Autodesk Inventor part; units mm, degrees
ref_plane "YZ Plane" through (0, 0, 0) normal (1, 0, 0) x (0, 1, 0)
ref_plane "XZ Plane" through (0, 0, 0) normal (0, 1, 0) x (-1, 0, 0)
ref_plane "XY Plane" through (0, 0, 0) normal (0, 0, 1) x (1, 0, 0)
sketch "Sketch1" plane through (0, 0, 0) normal (0, 0, 1) x (1, 0, 0)
  circle A0 centre (0, 0) radius 1.5
  arc A1 (-0.6702, -11.9813) -> (0, 12) centre (0, 0) ccw
  circle A2 centre (-50, 0) radius 1.5
  arc A3 (-6.6581, 4.4351) -> (-6.6581, -4.4351) centre (0, 0) ccw
  line L0 (-44.9603, 5.4977) -> (-8.4343, 7.5407)
  line L1 (-44.9603, -5.4977) -> (-8.4343, -7.5407)
  arc A4 (-44.9603, 5.4977) -> (-46.0589, 3.0769) centre (-44.8765, 4) ccw
  arc A5 (-46.0589, -3.0769) -> (-44.9603, -5.4977) centre (-44.8765, -4) ccw
  arc A6 (-6.6581, 4.4351) -> (-8.4343, 7.5407) centre (-8.3226, 5.5439) ccw
  arc A7 (-8.4343, -7.5407) -> (-6.6581, -4.4351) centre (-8.3226, -5.5439) ccw
  line L2 (-104, 0) -> (-57, 0) construction
  line L3 (-106, -18) -> (-104, -18)
  line L4 (-98, -12) -> (-98, -6.6741)
  line L5 (-112, -12) -> (-112, 18)
  arc A8 (-94.8953, -3.6759) -> (-98, -6.6741) centre (-95, -6.6741) ccw
  arc A9 (-106, 24) -> (-112, 18) centre (-106, 18) ccw
  arc A10 (-112, -12) -> (-106, -18) centre (-106, -12) ccw
  arc A11 (-104, -18) -> (-98, -12) centre (-104, -12) ccw
  arc A12 (-46.0589, -3.0769) -> (-46.0589, 3.0769) centre (-50, 0) ccw
  line L6 (-103, 19) -> (-106, -12) construction
  line L7 (-106.0856, 19.2986) -> (-109.0856, -11.7014)
  line L8 (-109.0856, -11.7014) -> (-102.9144, -12.2986)
  line L9 (-106.0856, 19.2986) -> (-99.9144, 18.7014)
  line L10 (-99.9144, 18.7014) -> (-102.9144, -12.2986)
  line L11 (-106, 24) -> (-103, 24)
  arc A13 (-98, 15) -> (-95, 12) centre (-95, 15) ccw
  line L12 (-95, 12) -> (-54, 12)
  line L13 (-47.8018, 9.3262) -> (0, 12)
  line L14 (-50.2234, -9.2095) -> (-0.6702, -11.9813)
  line L15 (-56.9088, -5.0024) -> (-94.8953, -3.6759)
  arc A14 (-51.0126, 10.66) -> (-54, 12) centre (-54, 8) ccw
  arc A15 (-51.0126, 10.66) -> (-47.8018, 9.3262) centre (-48.0252, 13.32) ccw
  arc A16 (-53.5242, -7.1079) -> (-50.2234, -9.2095) centre (-50, -5.2158) ccw
  arc A17 (-53.5242, -7.1079) -> (-56.9088, -5.0024) centre (-57.0484, -9) ccw
  line L16 (-91.3398, 7) -> (-58.0777, 7)
  line L17 (-59.5071, -0.9093) -> (-91.5071, 0.2082)
  line L18 (-93.4361, 2.2768) -> (-93.3386, 5.0698)
  arc A18 (-56.3772, 3.9474) -> (-57.4505, 0.8601) centre (-50, 0) ccw
  arc A19 (-59.5071, -0.9093) -> (-57.4505, 0.8601) centre (-59.4373, 1.0895) ccw
  arc A20 (-56.3772, 3.9474) -> (-58.0777, 7) centre (-58.0777, 5) ccw
  arc A21 (-91.3398, 7) -> (-93.3386, 5.0698) centre (-91.3398, 5) ccw
  arc A22 (-93.4361, 2.2768) -> (-91.5071, 0.2082) centre (-91.4373, 2.207) ccw
  line L19 (-98, 15) -> (-98, 19)
  arc A23 (-98, 19) -> (-103, 24) centre (-103, 19) ccw
  point P0 (-0.4468, -7.9875)
  point P1 (-94.8178, 5.6675)
  point P2 (-94.8178, 5.6675)
  point P3 (-52.6926, 7)
  point P4 (-57.4355, -0.9816)
  dimension "d0" = 3
  dimension "d2" = 12
  dimension "d10" = 50
  dimension "d14" = 16
  dimension "d18" = 2
  dimension "d31" = 7
  dimension "d42" = 3
  dimension "d43" = 6
  dimension "d52" = 14
  dimension "d53" = 98
  dimension "d57" = 18
  dimension "d60" = 24
  dimension "d61" = 3.1
  dimension "d63" = 5
  dimension "d77" = 8
  dimension "d80" = 4
  dimension "d81" = 4
  dimension "d82" = 4
  dimension "d83" = 4
  dimension "d84" = 1.5
  dimension "d85" = 9
  dimension "d86" = 4
  dimension "d87" = 8
  dimension "d88" = 178
  dimension "d90" = 5
  dimension "d91" = 4
  dimension "d92" = 7.5
  dimension "d93" = 2
  dimension "d94" = 2
  dimension "d95" = 32
  dimension "d96" = 5
extrude "Extrusion1" add sketch "Sketch1" along normal blind 5.85
properties part number "tipper_link_C"
The listing builds one solid part. Answer for the finished solid, in the listing's coordinates (mm). A direction names the side the tool comes from. Round coordinates to 2 decimals unless told otherwise and drop trailing zeros. Order: outer loops, then holes, each group sorted by start corner. A loop starts at its lowest first (then second) coordinate and runs counter-clockwise, first axis right, second up. Notation, with made-up numbers: (61, 35.25) -> (89, 35.25) arc R21 ccw to (89, 63.25) -> close; hole circle Ø6 at (29, -2.75). An arc over 180 degrees is marked (long way). Write each question's results on one line, items separated by ' | '. Start each with the question number.
Q1. The mould has two halves that part along Y. Classify faces 3 (the cylindrical face through (-57.09, 2.44, 2.88)), 4 (the cylindrical face through (-52.384, 11.659, 2.884)), 5 (the cylindrical face through (-52.12, -8.61, 2.88)), 6 (the flat face through (-112, 3, 3)): pulls with the +Y half, pulls with the -Y half, needs draft (parallel to the pull), parting line crosses it, or undercut.
Q2. Find section B-B (x = -26.5). Determine the outline of the cut face in (y, z), then the cut area to 3 significant figures.
Q3. Which of the six approach directions +Z, -Z, +X, -X, +Y, -Y give full straight-line access (tool end or side, diameter ignored) to faces 1 (the flat face through (-26.953, 6.505, 2.884)), 2 (the flat face through (-55, 0, 5.85))?
Q4. Find section A-A (y = -10.5). Determine the outline of the cut face in (x, z), then the cut area to 3 significant figures.
Q5. Straight lines are drawn through the part: probe 1 along X at (y, z) = (-1, 2.7); probe 2 along Y at (x, z) = (-7, 3.25); probe 3 along Y at (x, z) = (-105.5, 1.65). For each, find the intervals that lie inside material, in ascending order. Write a range as from..to.
Q6. Each of these flat-tipped pins is pushed along its axis until it touches: pin 1 (2 mm diameter, centred on y = 17, z = 2, fed in from +X); pin 2 (10 mm diameter, centred on x = -38, y = 18, fed in from -Z); pin 3 (2 mm diameter, centred on x = -13, z = 1.5, fed in from +Y); pin 4 (2.5 mm diameter, centred on y = -9, z = 2, fed in from +X). Where does it stop, or does it pass through?
Q7. Find section D-D (y = 21). Determine the outline of the cut face in (x, z).
Q8. Find section C-C (z = 1). Give the number of separate pieces and of enclosed holes in the cut face, then the cut area to 3 significant figures.
Worked answers:
1) face 3: undercut | face 4: pulls with the +Y half | face 5: pulls with the -Y half | face 6: needs draft
2) outline: (-10.54, 0) -> (-6.53, 0) -> (-6.53, 5.85) -> (-10.54, 5.85) -> close; (6.53, 0) -> (10.52, 0) -> (10.52, 5.85) -> (6.53, 5.85) -> close | area: 46.8 mm2
3) face 1: +Z, -Z | face 2: +Z, +X, -X, +Y, -Y
4) outline: (-112, 0) -> (-108.97, 0) -> (-108.97, 5.85) -> (-112, 5.85) -> close; (-102.74, 0) -> (-98, 0) -> (-98, 5.85) -> (-102.74, 5.85) -> close; (-27.15, 0) -> (5.81, 0) -> (5.81, 5.85) -> (-27.15, 5.85) -> close | area: 238 mm2
5) probe 1: x = -112..-108.05, -101.82..-51.12, -48.88..-45.1, -7.94..-1.12, 1.12..11.96 | probe 2: y = -11.63..-7.04, -3.87..3.87, 7.04..11.61 | probe 3: y = -18..-12.05, 19.24..24
6) pin 1: stops at x = -98 | pin 2: passes through | pin 3: stops at y = 11.33 | pin 4: stops at x = 9.16
7) outline: (-111.2, 0) -> (-98.42, 0) -> (-98.42, 5.85) -> (-111.2, 5.85) -> close
8) separate pieces: 1 | enclosed holes: 5 | area: 1,670 mm2
